from build123d import *

# Parameters (mm, degrees)
ESQUISSE1_W             = 45
ESQUISSE1_H             = 40
BOSS_EXTRU_1_DEPTH      = 8
ESQUISSE2_R             = 7.5
ENL_V_MAT_EXTRU_1_DEPTH = 9
ESQUISSE3_R             = 9.5
ENL_V_MAT_EXTRU_2_DEPTH = 6
ESQUISSE4_R             = 2
ENL_V_MAT_EXTRU_3_DEPTH = 41


with BuildPart() as part:
    # Esquisse1 → Boss.-Extru.1 (new body)
    with BuildSketch(Plane.XY):
        Rectangle(ESQUISSE1_W, ESQUISSE1_H)
    extrude(amount=BOSS_EXTRU_1_DEPTH)

    # Esquisse2 → Enlèv. mat.-Extru.1 (cut, through all)
    with BuildSketch(Plane.XY.offset(8)):
        Circle(ESQUISSE2_R)
    extrude(amount=-ENL_V_MAT_EXTRU_1_DEPTH, mode=Mode.SUBTRACT)

    # Esquisse3 → Enlèv. mat.-Extru.2 (cut)
    with BuildSketch(Plane.XY.offset(8)):
        Circle(ESQUISSE3_R)
    extrude(amount=-ENL_V_MAT_EXTRU_2_DEPTH, mode=Mode.SUBTRACT)

    # Esquisse4 → Enlèv. mat.-Extru.3 (cut, through all)
    with BuildSketch(Plane(origin=(0, 20, 0), x_dir=(1, 0, 0), z_dir=(0, 1, 0))):
        with Locations((-17.5, -4)):
            Circle(ESQUISSE4_R)
        with Locations((17.5, -4)):
            Circle(ESQUISSE4_R)
    extrude(amount=-ENL_V_MAT_EXTRU_3_DEPTH, mode=Mode.SUBTRACT)


solid = part.part
Here's how the part is built. I have some questions about the finished solid (model axes, mm). A direction names the side the tool comes from. Give positions to 0.01 mm unless a question says otherwise; leave off trailing zeros. Order: outer loops, then holes, each group sorted by start corner. A loop starts at its lowest first (then second) coordinate and runs counter-clockwise, first axis right, second up. Notation, with made-up numbers: (82.25, 81) -> (98.25, 81) arc R17 cw to (98.25, 102) -> close; hole circle Ø10 at (24, 15.25). An arc over 180 degrees is marked (long way). Use a Markdown table: item, result. Add a question column.
Item 1: Imagine slicing it at D-D on x = 0. Please give me the cut outline in (y, z).
Item 2: I need wall thicknesses on line 1 (X direction, y = -10.5, z = 4); line 2 (X direction, y = 1.5, z = 4); line 3 (X direction, y = 6.5, z = 4). Which ranges of each line are inside material? Lowest first, please.
Item 3: Imagine slicing it at C-C on z = 4. Please give me the cut outline in (x, y).
Item 4: Imagine slicing it at B-B on x = 17.5. Please give me the cut outline in (y, z), plus the area to 3 significant figures.
Item 5: For faces 5 (the face through (1, 8, 2)), 6 (the face through (-7.493, 0.33, 1.014)), which set-ups out of +Z, -Z, +X, -X, +Y, -Y let a thin tool reach every point of the face, with its end or its side?
Item 6: Imagine slicing it at A-A on y = 0. Please give me the cut outline in (x, z), plus the area to 3 significant figures.
Item 7: If we mould it in two halves opening along X, with no side actions, what happens to faces 1 (the face through (0, -20, 4)), 2 (the face through (4.38, -8.43, 5.04)), 3 (the face through (-22.5, 0, 4)), 4 (the face through (22.5, 0, 4))? For each: pulls with the +X half, pulls with the -X half, needs draft (parallel to the pull), parting line crosses it, or undercut.
Data:
| question | item | result |
|---|---|---|
| 1 | outline | (-20, 0) -> (-7.5, 0) -> (-7.5, 2) -> (-9.5, 2) -> (-9.5, 8) -> (-20, 8) -> close; (7.5, 0) -> (20, 0) -> (20, 8) -> (9.5, 8) -> (9.5, 2) -> (7.5, 2) -> close |
| 2 | line 1 | x = -22.5 to -19.5, -15.5 to 15.5, 19.5 to 22.5 |
| 2 | line 2 | x = -22.5 to -19.5, -15.5 to -9.38, 9.38 to 15.5, 19.5 to 22.5 |
| 2 | line 3 | x = -22.5 to -19.5, -15.5 to -6.93, 6.93 to 15.5, 19.5 to 22.5 |
| 3 | outline | (-22.5, -20) -> (-19.5, -20) -> (-19.5, 20) -> (-22.5, 20) -> close; (-15.5, -20) -> (15.5, -20) -> (15.5, 20) -> (-15.5, 20) -> close; (19.5, -20) -> (22.5, -20) -> (22.5, 20) -> (19.5, 20) -> close; hole circle Ø19 at (0, 0) |
| 4 | outline | (-20, 0) -> (20, 0) -> (20, 2) -> (-20, 2) -> close; (-20, 6) -> (20, 6) -> (20, 8) -> (-20, 8) -> close |
| 4 | area | 160 mm² |
| 5 | face 5 | +Z |
| 5 | face 6 | +Z, -Z |
| 6 | outline | (-22.5, 0) -> (-7.5, 0) -> (-7.5, 2) -> (-9.5, 2) -> (-9.5, 8) -> (-22.5, 8) -> close; (7.5, 0) -> (22.5, 0) -> (22.5, 8) -> (9.5, 8) -> (9.5, 2) -> (7.5, 2) -> close; hole circle Ø4 at (-17.5, 4); hole circle Ø4 at (17.5, 4) |
| 6 | area | 191 mm² |
| 7 | face 1 | needs draft |
| 7 | face 2 | undercut |
| 7 | face 3 | pulls with the -X half |
| 7 | face 4 | pulls with the +X half |
